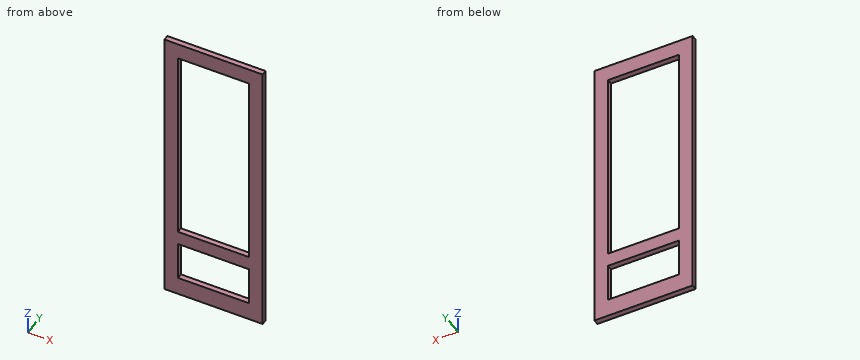
from build123d import *

# Parameters (mm, degrees)
F0_W          = 806.45
F0_H          = 2413
F0_W_2        = 584.2
F0_H_2        = 317.5
F0_H_3        = 1625.6
F1_DEPTH      = 22.225
F1_DEPTH_BACK = 22.225
F2_W          = 1248.5843106929
F2_H          = 271.0993243682
F2_H_2        = 504.0157202398
F3_DEPTH      = 22.226
F3_DEPTH_BACK = 22.226


# Not quite as in the source:
# - a length typed as a fraction of an inch, garbled in the dataset ("3 / 203.2 mm" for 3/8 in), is restored


with BuildPart() as f1:
    # F0 (on Front) → F1 (new body, two sides)
    with BuildSketch(Plane.XZ) as f1_sk:
        Rectangle(F0_W, F0_H)
        with Locations((0, -822.325)):
            Rectangle(F0_W_2, F0_H_2, mode=Mode.SUBTRACT)
        with Locations((0, 263.525)):
            Rectangle(F0_W_2, F0_H_3, mode=Mode.SUBTRACT)
    extrude(amount=F1_DEPTH)
    extrude(f1_sk.sketch, amount=-F1_DEPTH_BACK)

    # F2 (on Front) → F3 (cut, two sides)
    with BuildSketch(Plane.XZ) as f3_sk:
        with Locations((62.8663003445, 1342.0496621841)):
            Rectangle(F2_W, F2_H)
        with Locations((62.8663003445, -1382.3078601199)):
            Rectangle(F2_W, F2_H_2)
    extrude(amount=-F3_DEPTH, mode=Mode.SUBTRACT)
    extrude(f3_sk.sketch, amount=F3_DEPTH_BACK, mode=Mode.SUBTRACT)


solid = f1.part
Work out the finished part from the listing and answer in its coordinate system (mm). Give positions to 0.01 mm unless a question says otherwise; leave off trailing zeros. Loops run counter-clockwise (first coordinate to the right, second up) from the corner with the lowest first, then second, coordinate; pieces in that order, holes last. Notation, with made-up numbers: (47, 88) -> (88, 88) arc R19 ccw to (88, 111) -> close; hole circle Ø8 at (-38.5, -25). An arc over 180 degrees is marked (long way). Use a Markdown table: item, result. Add a question column.
1) The part is cut by section A-A, the plane x = 207. Determine the outline of the cut face in (y, z) (3 decimals).
2) The part is cut by section C-C, the plane y = 2. Determine the outline of the cut face in (x, z) (3 decimals), plus the area to 3 significant figures.
3) Consider line 1 along Z through (x, y) = (274.5, -14) (3 decimals); line 2 along X through (y, z) = (-14.5, -878) (3 decimals). Determine where each line is inside the solid, lowest interval first.
4) The part is cut by section B-B, the plane z = -424. Determine the outline of the cut face in (x, y) (3 decimals).
Reported:
| question | item | result |
|---|---|---|
| 1 | outline | (-22.225, -1130.3) -> (22.225, -1130.3) -> (22.225, -981.075) -> (-22.225, -981.075) -> close; (-22.225, -663.575) -> (22.225, -663.575) -> (22.225, -549.275) -> (-22.225, -549.275) -> close; (-22.225, 1076.325) -> (22.225, 1076.325) -> (22.225, 1206.5) -> (-22.225, 1206.5) -> close |
| 2 | outline | (-403.225, -1130.3) -> (403.225, -1130.3) -> (403.225, 1206.5) -> (-403.225, 1206.5) -> close; hole (-292.1, -981.075) -> (292.1, -981.075) -> (292.1, -663.575) -> (-292.1, -663.575) -> close; hole (-292.1, -549.275) -> (292.1, -549.275) -> (292.1, 1076.325) -> (-292.1, 1076.325) -> close |
| 2 | area | 749,000 mm^2 |
| 3 | line 1 | z = -1130.3 to -981.075, -663.575 to -549.275, 1076.325 to 1206.5 |
| 3 | line 2 | x = -403.225 to -292.1, 292.1 to 403.225 |
| 4 | outline | (-403.225, -22.225) -> (-292.1, -22.225) -> (-292.1, 22.225) -> (-403.225, 22.225) -> close; (292.1, -22.225) -> (403.225, -22.225) -> (403.225, 22.225) -> (292.1, 22.225) -> close |
